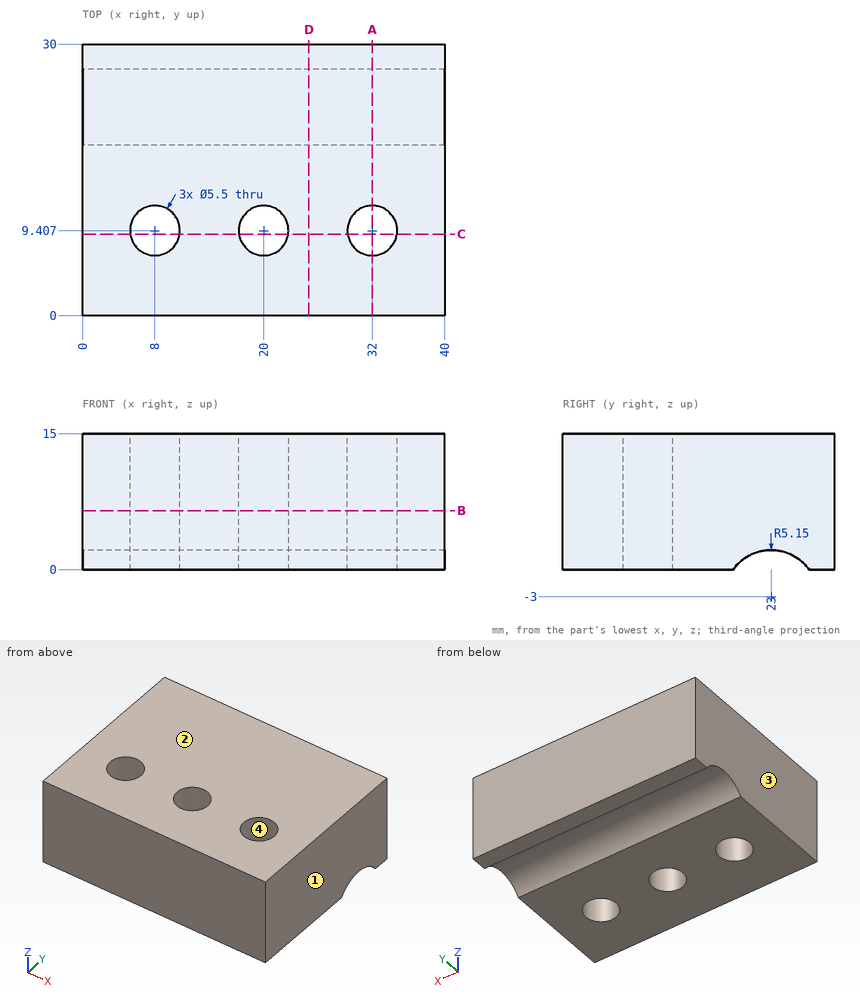
Design review of the part shown in the three views and the two pictorial views. Dimensions are in mm from the part's minimum x, y and z. Round coordinates to 2 decimals unless told otherwise and drop trailing zeros. Write each loop counter-clockwise with the first axis right and the second up, starting at its lowest first coordinate (ties: lowest second). Pieces come first, ordered by that corner, then holes. Notation, with made-up numbers: (50, 87) - (60, 87) arc R19 ccw to (60, 114) - close; hole circle Ø10 at (25, 48). An arc over 180 degrees is marked (long way). Answer as CSV lines item,"result". Start each with the question number.
(1) Add section D-D, the plane x = 25. State the section outline as (y, z) points, plus the area to 3 significant figures.
(2) For pin 1 (1 mm diameter, centred on x = 13.5, z = 6.5, fed in from -Y), flat-tipped, find the tip position at first contact; note if it passes through.
(3) Add section B-B, the plane z = 6.5. State the section outline as (x, y) points.
(4) Mouldability with a two-part tool opening along X and no side actions: class the marked faces 1, 2, 3 and 4 as +X half, -X half, draft (parallel to the pull), parting line (faces both ways), or undercut.
(5) Add section A-A, the plane x = 32. State the section outline as (y, z) points, plus the area to 3 significant figures.
(6) For line 1 (Y direction, x = 20, z = 8); line 2 (X direction, y = 11.5, z = 2.75); line 3 (X direction, y = 10.5, z = 5.75), list the stretches that pass through material, from the lowest coordinate up.
(7) Add section C-C, the plane y = 9. State the section outline as (x, z) points.
From the geometry:
1,outline,"(0, 0) - (18.81, 0) arc R5.15 cw to (27.19, 0) - (30, 0) - (30, 15) - (0, 15) - close"
1,area,"437 mm²"
2,pin 1,"stops at y = 0"
3,outline,"(0, 0) - (40, 0) - (40, 30) - (0, 30) - close; hole circle Ø5.5 at (8, 9.41); hole circle Ø5.5 at (20, 9.41); hole circle Ø5.5 at (32, 9.41)"
4,face 1,"+X half"
4,face 2,"draft"
4,face 3,"-X half"
4,face 4,"undercut"
5,outline,"(0, 0) - (6.66, 0) - (6.66, 15) - (0, 15) - close; (12.16, 0) - (18.81, 0) arc R5.15 cw to (27.19, 0) - (30, 0) - (30, 15) - (12.16, 15) - close"
5,area,"355 mm²"
6,line 1,"y = 0 to 6.66, 12.16 to 30"
6,line 2,"x = 0 to 6.22, 9.78 to 18.22, 21.78 to 30.22, 33.78 to 40"
6,line 3,"x = 0 to 5.48, 10.52 to 17.48, 22.52 to 29.48, 34.52 to 40"
7,outline,"(0, 0) - (5.28, 0) - (5.28, 15) - (0, 15) - close; (10.72, 0) - (17.28, 0) - (17.28, 15) - (10.72, 15) - close; (22.72, 0) - (29.28, 0) - (29.28, 15) - (22.72, 15) - close; (34.72, 0) - (40, 0) - (40, 15) - (34.72, 15) - close"
